Source: CAD feature listing. Evaluate the final solid. Frame: model axes, mm. Face numbers are marked on the shaded views. Coordinates: 2 decimals unless noted, no trailing zeros. Order: outer loops, then holes, each group sorted by start corner. A loop starts at its lowest first (then second) coordinate and runs counter-clockwise, first axis right, second up.
Item 1: Section D-D on y = 18.5. Return the cut outline in (x, z), then the cut area to 3 significant figures.
Item 2: Contact query for flat-ended pins moving along their axis: P1, Ø2.5, axis at y = 4, z = 6.5, coming from the +X side; P2, Ø5, axis at x = -3.5, z = 3, coming from the +Y side; P3, Ø4.5, axis at x = -3, y = 17.5, coming from the +Z side. Output: stop coordinate, or through.
Item 3: Section C-C on x = 0. Return the cut outline in (y, z).
Item 4: Mould query, pull axis X, two halves, no side actions, for the marked faces 1, 2, 3 and 4. Classes: released by +X, released by -X, zero draft, split by the parting line, or undercut.
Item 5: Section A-A on y = 2.5. Return the cut outline in (x, z), then the cut area to 3 significant figures.
Item 6: Section B-B on z = 1.75. Return the cut outline in (x, y), then the cut area to 3 significant figures.
Item 7: Ray query, line 1 (Y direction, x = 2.75, z = 6.5); line 2 (Z direction, x = 2.2, y = 2.5); line 3 (Y direction, x = 0, z = 3.7). Return the intervals inside material, ascending.
from build123d import *

# Parameters (mm, degrees)
EXTRUDE_1_DEPTH     = 4
CUT_EXTRUDE_1_DEPTH = 3
SKETCH_5_R          = 1.25
CUT_EXTRUDE_2_DEPTH = 12.4
SKETCH_6_W          = 1
SKETCH_6_H          = 10
CUT_EXTRUDE_3_DEPTH = 16.3
SKETCH_9_W          = 5
SKETCH_9_H          = 10
EXTRUDE_4_DEPTH     = 3
SKETCH_10_R         = 1.25
CUT_EXTRUDE_4_DEPTH = 5.1


with BuildPart() as part:
    # 草圖1 → 填料-伸長1 (new body)
    with BuildSketch(Plane.XY):
        with BuildLine():
            Line((7.5, 0), (7.5, 52))
            ThreePointArc((7.5, 52), (0, 59.5), (-7.5, 52))
            Line((-7.5, 52), (-7.5, 0))
            Line((-7.5, 0), (7.5, 0))
        make_face()
    extrude(amount=EXTRUDE_1_DEPTH)

    # 草圖3 → 除料-伸長1 (cut)
    with BuildSketch(Plane.XY):
        with BuildLine():
            ThreePointArc((-2.296635758, 50), (0, 52.296635758), (2.296635758, 50))
            Line((2.296635758, 50), (5, 33.5))
            Line((5, 33.5), (2.272331993, 16.632537074))
            ThreePointArc((2.272331993, 16.632537074), (-0.184323371, 14.705540024), (-2.301851795, 17))
            Line((-2.301851795, 17), (-5, 33.5))
            Line((-5, 33.5), (-2.296635758, 50))
        make_face()
    extrude(amount=CUT_EXTRUDE_1_DEPTH, mode=Mode.SUBTRACT)

    # 草圖5 → 除料-伸長2 (cut)
    with BuildSketch(Plane.XY):
        with Locations((0, 33.5)):
            Circle(SKETCH_5_R)
    extrude(amount=CUT_EXTRUDE_2_DEPTH, mode=Mode.SUBTRACT)

    # 草圖6 → 除料-伸長3 (cut)
    with BuildSketch(Plane.XY):
        with Locations((0, 5)):
            Rectangle(SKETCH_6_W, SKETCH_6_H)
    extrude(amount=CUT_EXTRUDE_3_DEPTH, mode=Mode.SUBTRACT)

    # 草圖9 → 填料-伸長4 (add)
    with BuildSketch(Plane(origin=(0.5, 0, 0), x_dir=(0, 0, -1), z_dir=(1, 0, 0))):
        with Locations((-6.46178466, 5)):
            Rectangle(SKETCH_9_W, SKETCH_9_H)
    extrude(amount=EXTRUDE_4_DEPTH)

    # 草圖10 → 除料-伸長4 (cut)
    with BuildSketch(Plane(origin=(0.5, 0, 0), x_dir=(0, 0, -1), z_dir=(1, 0, 0))):
        with Locations((-6.48089233, 7.5)):
            Circle(SKETCH_10_R)
        with Locations((-6.48089233, 2.5)):
            Circle(SKETCH_10_R)
    extrude(amount=CUT_EXTRUDE_4_DEPTH, mode=Mode.SUBTRACT)


solid = part.part
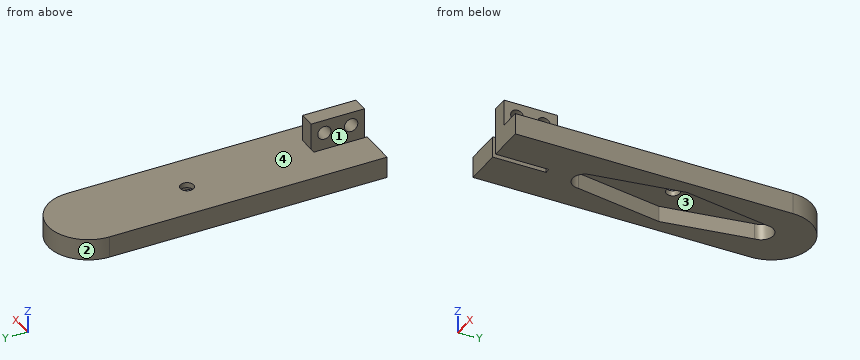
Answer list:
1. outline: (-7.5, 0) - (-2.55, 0) - (-2.55, 3) - (2.57, 3) - (2.57, 0) - (7.5, 0) - (7.5, 4) - (-7.5, 4) - close
1. area: 44.6 mm2
2. P1: stops at x = 3.5
2. P2: stops at y = 59.43
2. P3: stops at z = 4
3. outline: (10, 0) - (14.7, 0) - (14.7, 3) - (32.25, 3) - (32.25, 4) - (10, 4) - close; (34.75, 3) - (52.3, 3) - (52.3, 0) - (59.5, 0) - (59.5, 4) - (34.75, 4) - close
4. face 1: undercut
4. face 2: split by the parting line
4. face 3: undercut
4. face 4: zero draft
5. outline: (-7.5, 0) - (-0.5, 0) - (-0.5, 4) - (-7.5, 4) - close; (0.5, 0) - (7.5, 0) - (7.5, 4) - (3.5, 4) - (3.5, 5.23) - (0.5, 5.23) - close; (0.5, 7.73) - (3.5, 7.73) - (3.5, 8.96) - (0.5, 8.96) - close
5. area: 63.4 mm2
6. outline: (-7.5, 0) - (-0.5, 0) - (-0.5, 10) - (0.5, 10) - (0.5, 0) - (7.5, 0) - (7.5, 52) arc R7.5 ccw to (-7.5, 52) - close; hole (-5, 33.5) - (-2.3, 17) arc R2.3 ccw to (2.27, 16.63) - (5, 33.5) - (2.3, 50) arc R2.3 ccw to (-2.3, 50) - close
6. area: 601 mm2
7. line 1: y = 0 to 1.25, 3.75 to 6.25, 8.75 to 10
7. line 2: z = 0 to 5.23, 7.73 to 8.96
7. line 3: y = 10 to 32.25, 34.75 to 59.5
